from build123d import *
from build123d.topology import SkipClean

# Parameters (mm, degrees)
CROQUIS1_R              = 21
SALIENTE_EXTRUIR1_DEPTH = 40
SALIENTE_EXTRUIR2_DEPTH = 40
SALIENTE_EXTRUIR3_REACH = 77.493
CROQUIS3_R              = 13.5
CROQUIS3_R_2            = 10
CROQUIS7_R              = 8.227269221
CROQUIS7_R_2            = 6
CORTAR_EXTRUIR6_DEPTH   = 6
CROQUIS8_R              = 6
CORTAR_EXTRUIR7_DEPTH   = 72.223648425
CORTAR_EXTRUIR8_START   = -25
CORTAR_EXTRUIR8_DEPTH   = 25
CROQUIS12_R             = 9.55
CORTAR_EXTRUIR9_DEPTH   = 5.5
CORTAR_EXTRUIR10_DEPTH  = 72.223648425


with BuildPart() as part:
    # Croquis1 → Saliente-Extruir1 (new body)
    with BuildSketch(Plane(origin=(0, 0, 0), x_dir=(1, 0, 0), z_dir=(0, 1, 0))):
        with Locations(Location((0, 0, 0), (0, 0, 270))):
            Circle(CROQUIS1_R)
    extrude(amount=SALIENTE_EXTRUIR1_DEPTH)

    # Croquis2 → Saliente-Extruir2 (add)
    with BuildSketch(Plane(origin=(0, 0, 0), x_dir=(1, 0, 0), z_dir=(0, 1, 0))):
        with BuildLine():
            Line((53.975127576, 8.110971331), (53.975127576, -11.889028669))
            Line((53.975127576, -11.889028669), (3.613793412, -20.686722727))
            ThreePointArc((3.613793412, -20.686722727), (20.98607707, -0.764571273), (5.109545014, 20.368911354))
            Line((5.109545014, 20.368911354), (53.975127576, 8.110971331))
        make_face()
    extrude(amount=SALIENTE_EXTRUIR2_DEPTH)

    # Croquis3 → Saliente-Extruir3 (add, up to next)
    with BuildSketch(Plane(origin=(5.109545014, 0, -20.368911354), x_dir=(-0.9699481597219111, 0, -0.24331166731597212), z_dir=(0.2433116673159721, 0, -0.969948159721911)), mode=Mode.PRIVATE) as saliente_extruir3_sk1:
        with Locations((0, 20)):
            Circle(CROQUIS3_R)
        with Locations((0, 20)):
            Circle(CROQUIS3_R_2, mode=Mode.SUBTRACT)
    saliente_extruir3_tool1 = extrude(saliente_extruir3_sk1.sketch, amount=-SALIENTE_EXTRUIR3_REACH, mode=Mode.PRIVATE) - part.part
    add(saliente_extruir3_tool1.solids().sort_by_distance((17.833482, 20, -17.177109))[0])

    # Croquis7 → Cortar-Extruir6 (cut)
    with BuildSketch(Plane.XZ):
        with Locations(Location((0, 0, 0), (0, 0, 270))):
            Circle(CROQUIS7_R)
        with Locations(Location((0, 0, 0), (0, 0, 270))):
            Circle(CROQUIS7_R_2, mode=Mode.SUBTRACT)
    extrude(amount=-CORTAR_EXTRUIR6_DEPTH, mode=Mode.SUBTRACT)

    # Croquis8 → Cortar-Extruir7 (cut, through all)
    with BuildSketch(Plane.XZ):
        with Locations(Location((0, 0, 0), (0, 0, 270))):
            Circle(CROQUIS8_R)
    extrude(amount=-CORTAR_EXTRUIR7_DEPTH, mode=Mode.SUBTRACT)

    # Croquis10 → Cortar-Extruir8 (cut)
    with BuildSketch(Plane(origin=(0, 40, 0), x_dir=(1, 0, 0), z_dir=(0, 1, 0)).offset(CORTAR_EXTRUIR8_START)):
        with BuildLine():
            Line((-5.995438853, 0.23390802), (-11.37823559, 0.424457107))
            Line((-11.37823559, 0.424457107), (-11.767631672, -10.575542893))
            Line((-11.767631672, -10.575542893), (30.232368328, -12.062327932))
            Line((30.232368328, -12.062327932), (30.62176441, -1.062327932))
            Line((30.62176441, -1.062327932), (5.996971268, -0.190619027))
            ThreePointArc((5.996971268, -0.190619027), (-0.212264906, -5.996244125), (-5.995438853, 0.23390802))
        make_face()
        with BuildLine():
            Line((-10.988839509, 11.424457107), (-11.37823559, 0.424457107))
            Line((-11.37823559, 0.424457107), (-5.995438853, 0.23390802))
            ThreePointArc((-5.995438853, 0.23390802), (0.116976243, 5.998859605), (6, 0))
            ThreePointArc((6, 0), (5.999242769, -0.095321543), (5.996971268, -0.190619027))
            Line((5.996971268, -0.190619027), (30.62176441, -1.062327932))
            Line((30.62176441, -1.062327932), (31.011160491, 9.937672068))
            Line((31.011160491, 9.937672068), (-10.988839509, 11.424457107))
        make_face()
    extrude(amount=CORTAR_EXTRUIR8_DEPTH, mode=Mode.SUBTRACT)

    # Croquis12 → Cortar-Extruir9 (cut)
    with BuildSketch(Plane(origin=(0, 15, 0), x_dir=(1, 0, 0), z_dir=(0, 1, 0))):
        with Locations(Location((0, 0, 0), (0, 0, 270))):
            Circle(CROQUIS12_R)
    extrude(amount=-CORTAR_EXTRUIR9_DEPTH, mode=Mode.SUBTRACT)

    # Croquis17 → Cortar-Extruir10 (cut, through all)
    with BuildSketch(Plane(origin=(0, 40, 0), x_dir=(1, 0, 0), z_dir=(0, 1, 0))):
        with BuildLine():
            Line((5.109545014, 20.368911354), (5.109545014, 31.680559043))
            Line((5.109545014, 31.680559043), (-13.688349404, 31.680559043))
            Line((-13.688349404, 31.680559043), (-13.688349404, 15.925736736))
            ThreePointArc((-13.688349404, 15.925736736), (-4.830571536, 20.436868122), (5.109545014, 20.368911354))
        make_face()
    extrude(amount=-CORTAR_EXTRUIR10_DEPTH, mode=Mode.SUBTRACT)

    # Croquis4 → Revolución1 (revolve)
    with SkipClean():  # the faces are left unmerged after this step: merging them gives an invalid solid
        with BuildSketch(Plane(origin=(5.1, 0, 0), x_dir=(0, 0, -1), z_dir=(1, 0, 0))):
            Polygon((13.998733147, 5.708275528), (49.038401492, 13.163524112), (49.038401492, 16.663524112), (20.838401492, 10.663524112), (13.998733147, 9.208275528), align=None)
        revolve(axis=Axis((5.1, 20.663524112, -20.838401492), (0, 0.20810764446485977, -0.9781059289848353)))


solid = part.part
Geometry check sheet. Reference: the model listing, model coordinates, mm. A direction names the side the tool comes from. Give positions to 0.01 mm unless a question says otherwise; leave off trailing zeros. Order: outer loops, then holes, each group sorted by start corner. A loop starts at its lowest first (then second) coordinate and runs counter-clockwise, first axis right, second up.
1. Sectioned sample at A-A (z = 5). Record the boundary of the cut face in (x, y).
Completed:
outline: (-20.4, 0) - (-6.53, 0) - (-6.53, 6) - (-3.32, 6) - (-3.32, 9.5) - (-8.14, 9.5) - (-8.14, 15) - (-11.57, 15) - (-11.57, 40) - (-20.4, 40) - close; (3.32, 6) - (6.53, 6) - (6.53, 0) - (53.98, 0) - (53.98, 40) - (30.48, 40) - (30.48, 15) - (8.14, 15) - (8.14, 9.5) - (3.32, 9.5) - close
2. Scan lines: line 1 (X direction, y = 12, z = 0); line 2 (X direction, y = 26.5, z = -27); line 3 (Y direction, x = -0.5, z = -11). Record each from-to range of solid material in increasing order.
Completed:
line 1: x = -21 to -9.55, 9.55 to 53.98
line 2: x = -7.34 to -3.62, 13.82 to 17.54
line 3: y = 0 to 15, 26.77 to 30.8
3. Draft check along X on faces 1 (the face through (4.66, 35.94, -44.9)), 2 (the face through (34.63, 19.72, -12.964)), 3 (the face through (8.841, 20.417, -19.433)), 4 (the face through (17, 0, 0)). Enter one of: pulls with the +X half, pulls with the -X half, needs draft (parallel to the pull), parting line crosses it, or undercut.
Completed:
face 1: parting line crosses it
face 2: pulls with the +X half
face 3: undercut
face 4: needs draft
4. Sectioned sample at B-B (x = 22). Record the boundary of the cut face in (y, z), then the cut area to 3 significant figures.
Completed:
outline: (0, -16.13) - (40, -16.13) - (40, -10.26) - (15, -10.26) - (15, 11.77) - (40, 11.77) - (40, 17.47) - (0, 17.47) - close
area: 794 mm2
5. Depth check by flat-ended pin: pin 1 (1 mm diameter, centred on x = 10, z = -38.5, fed in from +Y); pin 2 (21 mm diameter, centred on x = 0, z = -3.5, fed in from +Y); pin 3 (2 mm diameter, centred on x = 13, z = 4, fed in from +Y); pin 4 (6 mm diameter, centred on x = 12.5, z = -26, fed in from -Y). Enter the tip coordinate at first touch or a pass-through.
Completed:
pin 1: stops at y = 37.18
pin 2: stops at y = 40
pin 3: stops at y = 15
pin 4: stops at y = 8.87
6. Sectioned sample at C-C (x = 49). Record the boundary of the cut face in (y, z), then the cut area to 3 significant figures.
Completed:
outline: (0, -9.36) - (40, -9.36) - (40, 12.76) - (0, 12.76) - close
area: 885 mm2
7. Access from +Z, -Z, +X, -X, +Y, -Y to the whole of each face (thin tool, end or side, straight path). Record for faces 5 (the face through (-5, 6, -4)), 6 (the face through (17, 40, 14)), 7 (the face through (3.227, 28.369, -9.875)).
Completed:
face 5: -Y
face 6: +Z, -Z, +X, -X, +Y
face 7: none
